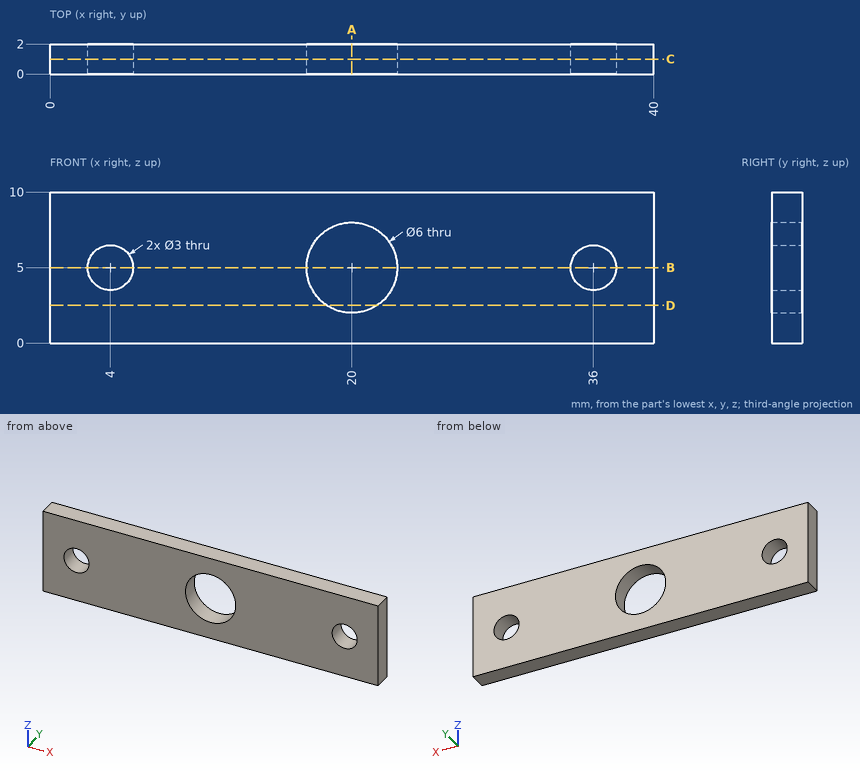
Could you check a few things on this drawing? It's one solid part, dimensions in mm from its lowest x, y, z. Coordinates: 2 decimals unless noted, no trailing zeros. Write each loop counter-clockwise with the first axis right and the second up, starting at its lowest first coordinate (ties: lowest second). Pieces come first, ordered by that corner, then holes. Notation, with made-up numbers: (87, 31) - (123, 31) arc R15 ccw to (123, 43) - close; hole circle Ø10 at (-37, -12). An arc over 180 degrees is marked (long way). Use one line per item in the form item = value.
1) I'm going to push a flat-ended pin straight in: P1, Ø1, axis at x = 10, y = 1.5, coming from the -Z side. Where does the tip first touch, or does it pass through?
Solved:
P1 = 0
2) Suppose I cut it at D-D, the plane z = 2.5. Write out the boundary of the cut face in (x, y), plus the area to 3 significant figures.
Solved:
outline = (0, 0) - (18.34, 0) - (18.34, 2) - (0, 2) - close; (21.66, 0) - (40, 0) - (40, 2) - (21.66, 2) - close
area = 73.4 mm2
3) Suppose I cut it at B-B, the plane z = 5. Write out the boundary of the cut face in (x, y).
Solved:
outline = (0, 0) - (2.5, 0) - (2.5, 2) - (0, 2) - close; (5.5, 0) - (17, 0) - (17, 2) - (5.5, 2) - close; (23, 0) - (34.5, 0) - (34.5, 2) - (23, 2) - close; (37.5, 0) - (40, 0) - (40, 2) - (37.5, 2) - close
4) I need wall thicknesses on line 1 (X direction, y = 0.8, z = 5); line 2 (X direction, y = 1.4, z = 5.5); line 3 (Z direction, x = 4, y = 0.5). Which ranges of each line are inside material? Lowest first, please.
Solved:
line_1 = 0 to 2.5, 5.5 to 17, 23 to 34.5, 37.5 to 40
line_2 = 0 to 2.59, 5.41 to 17.04, 22.96 to 34.59, 37.41 to 40
line_3 = 0 to 3.5, 6.5 to 10
5) Suppose I cut it at A-A, the plane x = 20. Write out the boundary of the cut face in (y, z), plus the area to 3 significant figures.
Solved:
outline = (0, 0) - (2, 0) - (2, 2) - (0, 2) - close; (0, 8) - (2, 8) - (2, 10) - (0, 10) - close
area = 8.00 mm2
6) Suppose I cut it at C-C, the plane y = 1. Write out the boundary of the cut face in (x, z).
Solved:
outline = (0, 0) - (40, 0) - (40, 10) - (0, 10) - close; hole circle Ø3 at (4, 5); hole circle Ø6 at (20, 5); hole circle Ø3 at (36, 5)
